Design review of the part built by this model. Coordinates are the model's own, in mm. Face numbers are marked on the shaded views. Coordinates: 2 decimals unless noted, no trailing zeros. Write each loop counter-clockwise with the first axis right and the second up, starting at its lowest first coordinate (ties: lowest second). Pieces come first, ordered by that corner, then holes.
Q1. Insertion check: pin 1 (4 mm diameter, centred on x = -34.5, y = 3.5, fed in from +Z); pin 2 (6 mm diameter, centred on x = 28, y = -6, fed in from +Z); pin 3 (1.5 mm diameter, centred on y = -6, z = 7.5, fed in from +X). Each pin has a flat end and moves straight along its axis. Give the tip position at first contact, or say it passes through.
Q2. Take a section at A-A (x = -12). Give the boundary of the cut face in (y, z), and give its area (3 significant figures).
Q3. Mouldability with a two-part tool opening along X and no side actions: class the marked faces 1 and 2 as pulls with the +X half, pulls with the -X half, needs draft (parallel to the pull), parting line crosses it, or undercut.
Q4. For probe 1 along X at (y, z) = (-6.75, 1.5); probe 2 along Y at (x, z) = (-27.5, 6.5); probe 3 along X at (y, z) = (-6.25, 0), list the stretches that pass through material, from the lowest coordinate up.
Q5. Take a section at B-B (x = 1). Give the boundary of the cut face in (y, z), and give its area (3 significant figures).
```python
from build123d import *


with BuildPart() as f1:
    # F0 (on Front) → F1 (revolve)
    with BuildSketch(Plane.XZ):
        with BuildLine():
            Line((-48.178779, 0), (-40.178779, 0))
            Line((-40.178779, 0), (43.821221, 0))
            Line((43.821221, 0), (46.321221, 0))
            Line((46.321221, 0), (64.321221, 0))
            ThreePointArc((64.321221, 0), (57.483499, 9.486833), (46.321221, 6))
            Line((46.321221, 6), (43.821221, 6))
            Line((43.821221, 6), (41.980936, 7.278439))
            ThreePointArc((41.980936, 7.278439), (37.367955, 12.34431), (30.734845, 14.060264))
            Line((30.734845, 14.060264), (-39.811072, 11.49412))
            ThreePointArc((-39.811072, 11.49412), (-43.994925, 13.5), (-48.178779, 11.49412))
            Line((-48.178779, 11.49412), (-48.178779, 0))
        make_face()
    revolve(axis=Axis((1.821221, 0, 0), (1, 0, 0)))


solid = f1.part
```
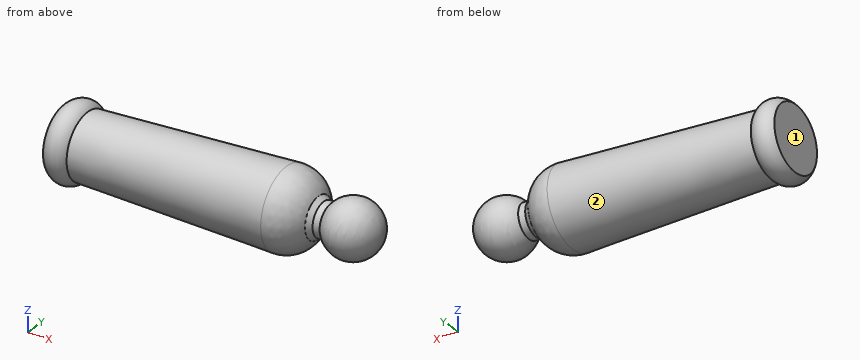
Response:
1. pin 1: stops at z = 11.6
1. pin 2: stops at z = 13.64
1. pin 3: stops at x = 58.97
2. outline: circle Ø25.01 at (0, 0)
2. area: 491 mm2
3. face 1: pulls with the -X half
3. face 2: undercut
4. probe 1: x = -48.18 to 42.5, 47.1 to 61.55
4. probe 2: y = -10.02 to 10.02
4. probe 3: x = -48.18 to 43.46, 46.51 to 62.13
5. outline: circle Ø25.96 at (0, 0)
5. area: 529 mm2
